Input: part model. Units: mm. Frame: model coordinates. Face numbers are marked on the shaded views. A direction names the side the tool comes from. Give positions to 0.01 mm unless a question says otherwise; leave off trailing zeros. Loops run counter-clockwise (first coordinate to the right, second up) from the corner with the lowest first, then second, coordinate; pieces in that order, holes last. Notation, with made-up numbers: M 69,3 L 101,3 A24 ccw 101,22 Z; hole C 10,-29.5 d9. An arc over 180 degrees is marked long. Use a Markdown table: item, result. Add a question column.
from build123d import *

# Parameters (mm, degrees)
SKETCH1_R           = 7
BOSS_EXTRUDE1_DEPTH = 7
SKETCH2_R           = 6
BOSS_EXTRUDE2_DEPTH = 33
CHAMFER1_SIZE       = 1


with BuildPart() as part:
    # Sketch1 → Boss-Extrude1 (new body)
    with BuildSketch(Plane.XY):
        Circle(SKETCH1_R)
    extrude(amount=BOSS_EXTRUDE1_DEPTH)

    # Sketch2 → Boss-Extrude2 (add)
    with BuildSketch(Plane.XY.offset(7)):
        Circle(SKETCH2_R)
    extrude(amount=BOSS_EXTRUDE2_DEPTH)

    # Chamfer1
    chamfer1_edges = [part.edges().sort_by_distance(p)[0] for p in [
        (-6, 0, 40),
    ]]
    chamfer(chamfer1_edges, length=CHAMFER1_SIZE)


solid = part.part
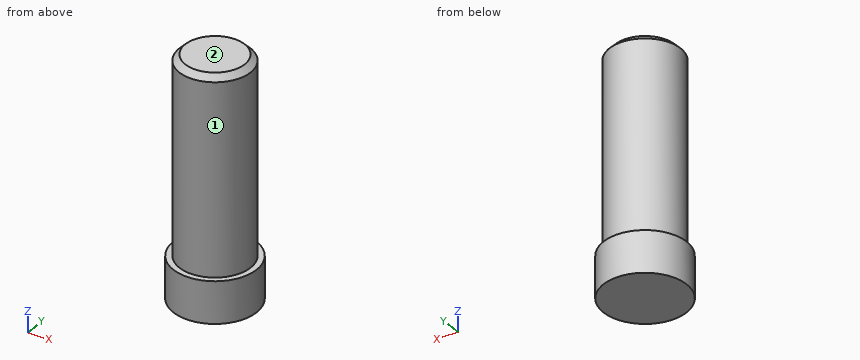
1) Contact query for flat-ended pins moving along their axis: P1, Ø8, axis at x = 0.5, z = 34.5, coming from the +Y side; P2, Ø2, axis at x = 4, y = 5.5, coming from the +Z side; P3, Ø1.5, axis at y = -2, z = 19.5, coming from the -X side. Output: stop coordinate, or through.
2) Section query A-A, the plane y = 0. Return the cut outline in (x, z), and give its area (3 significant figures).
3) Ray query, line 1 (Y direction, x = -2.5, z = 33.5); line 2 (X direction, y = 5, z = 26.5). Return the intervals inside material, ascending. Write a range as [from, to].
4) Section query C-C, the plane z = 24. Return the cut outline in (x, y).
5) Reachability of the marked faces 1 and 2 from +Z, -Z, +X, -X, +Y, -Y: full face, straight path, thin tool, end or side. Return the list, or none.
Entries:
| question | item | result |
|---|---|---|
| 1 | P1 | stops at y = 6 |
| 1 | P2 | stops at z = 39.2 |
| 1 | P3 | stops at x = -5.87 |
| 2 | outline | M -7,0 L 7,0 L 7,7 L 6,7 L 6,39 L 5,40 L -5,40 L -6,39 L -6,7 L -7,7 Z |
| 2 | area | 493 mm² |
| 3 | line 1 | y = [-5.45, 5.45] |
| 3 | line 2 | x = [-3.32, 3.32] |
| 4 | outline | C 0,0 d12 |
| 5 | face 1 | +Z |
| 5 | face 2 | +Z, +X, -X, +Y, -Y |
